The listing builds one solid part. Answer for the finished solid, in the listing's coordinates (mm). A direction names the side the tool comes from. Round coordinates to 2 decimals unless told otherwise and drop trailing zeros. Write each loop counter-clockwise with the first axis right and the second up, starting at its lowest first coordinate (ties: lowest second). Pieces come first, ordered by that corner, then holes.
from build123d import *

# Parameters (mm, degrees)
EXTRUDE1_DEPTH  = 4.7752
EXTRUDE2_DEPTH  = 12.938
SKETCH33_W      = 2.286
SKETCH33_H      = 5.588
EXTRUDE30_DEPTH = 10.668
EXTRUDE3_DEPTH  = 3.0988
EXTRUDE6_DEPTH  = 3.0988
EXTRUDE7_DEPTH  = 3.0988
SKETCH23_W      = 3.0988
SKETCH23_H      = 1.133450424
EXTRUDE20_DEPTH = 2.54
EXTRUDE16_DEPTH = 3.0988
FILLET1_R       = 0.762
EXTRUDE21_DEPTH = 3.0988
FILLET2_R       = 0.762
EXTRUDE28_DEPTH = 8.0612
EXTRUDE29_REACH = 9.061
FILLET3_R       = 0.762
FILLET4_R       = 0.508
FILLET5_R       = 0.508
FILLET6_R       = 0.508
SKETCH35_R      = 1.016
EXTRUDE32_DEPTH = 8.0612


with BuildPart() as part:
    # Sketch1 → Extrude1 (new body)
    with BuildSketch(Plane.XY):
        Polygon((-14.859, 11.938), (0, 11.938), (0, 4.572), (-3.175, 4.572), (-3.175, 0), (-14.859, 0), align=None)
    extrude(amount=-EXTRUDE1_DEPTH)

    # Sketch2 → Extrude2 (cut, through all)
    with BuildSketch(Plane(origin=(0, 11.938, 0), x_dir=(1, 0, 0), z_dir=(0, 1, 0))):
        Polygon((0, 0.5842), (-4.191, 4.7752), (0, 4.7752), align=None)
    extrude(amount=-EXTRUDE2_DEPTH, mode=Mode.SUBTRACT)

    # Sketch33 → Extrude30 (add)
    with BuildSketch(Plane.ZY.offset(14.859)):
        with Locations((-5.9182, 9.144)):
            Rectangle(SKETCH33_W, SKETCH33_H)
    extrude(amount=-EXTRUDE30_DEPTH)

    # Sketch5 → Extrude3 (cut)
    with BuildSketch(Plane.XY):
        with BuildLine():
            Line((-14.859, 8.121520088), (-14.859, 0))
            Line((-14.859, 0), (-8.374207602, 0))
            ThreePointArc((-8.374207602, 0), (-5.258197931, 4.182323512), (-8.261178378, 8.44652973))
            ThreePointArc((-8.261178378, 8.44652973), (-10.099280239, 8.911418564), (-11.9888, 9.0678))
            ThreePointArc((-11.9888, 9.0678), (-13.499883528, 8.825128765), (-14.859, 8.121520088))
        make_face()
    extrude(amount=-EXTRUDE3_DEPTH, mode=Mode.SUBTRACT)

    # Sketch8 → Extrude6 (add)
    with BuildSketch(Plane.XY):
        with BuildLine():
            Line((-5.916117419, 6.569687461), (-7.995771884, 6.569687461))
            ThreePointArc((-7.995771884, 6.569687461), (-8.381805974, 7.063274265), (-8.837117419, 7.493787609))
            Line((-8.837117419, 7.493787609), (-8.837117419, 8.601687461))
            ThreePointArc((-8.837117419, 8.601687461), (-7.16441835, 7.890723622), (-5.916117419, 6.569687461))
        make_face()
    extrude(amount=-EXTRUDE6_DEPTH)

    # Sketch9 → Extrude7 (add)
    with BuildSketch(Plane.XY):
        with BuildLine():
            Line((-5.916117419, 1.913912539), (-7.995771884, 1.913912539))
            ThreePointArc((-7.995771884, 1.913912539), (-8.381805974, 1.420325735), (-8.837117419, 0.989812391))
            Line((-8.837117419, 0.989812391), (-8.837117419, 0))
            Line((-8.837117419, 0), (-8.374207602, 0))
            ThreePointArc((-8.374207602, 0), (-6.971998867, 0.734557469), (-5.916117419, 1.913912539))
        make_face()
    extrude(amount=-EXTRUDE7_DEPTH)

    # Sketch23 → Extrude20 (add)
    with BuildSketch(Plane.ZY.offset(8.837117419)):
        with Locations((-1.5494, 8.060512821)):
            Rectangle(SKETCH23_W, SKETCH23_H)
    extrude(amount=-EXTRUDE20_DEPTH)

    # Sketch18 → Extrude16 (cut)
    with BuildSketch(Plane.XY):
        with BuildLine():
            Line((-4.903581733, 6.569687461), (-5.916117419, 6.569687461))
            ThreePointArc((-5.916117419, 6.569687461), (-5.2578, 4.2418), (-5.916117419, 1.913912539))
            Line((-5.916117419, 1.913912539), (-4.903581733, 1.913912539))
            ThreePointArc((-4.903581733, 1.913912539), (-4.3688, 4.2418), (-4.903581733, 6.569687461))
        make_face()
    extrude(amount=-EXTRUDE16_DEPTH, mode=Mode.SUBTRACT)

    # Fillet1
    fillet1_edges = [part.edges().sort_by_distance(p)[0] for p in [
        (0, 8.255, -0.5842),
    ]]
    fillet(fillet1_edges, radius=FILLET1_R)

    # Sketch24 → Extrude21 (add)
    with BuildSketch(Plane.XY):
        with BuildLine():
            Line((-8.837117419, 7.493787609), (-9.830149409, 8.301066631))
            ThreePointArc((-9.830149409, 8.301066631), (-10.843412246, 8.870424655), (-11.9888, 9.0678))
            Line((-11.9888, 9.0678), (-8.837117419, 9.0678))
            Line((-8.837117419, 9.0678), (-8.837117419, 7.493787609))
        make_face()
    extrude(amount=-EXTRUDE21_DEPTH)

    # Fillet2
    fillet2_edges = [part.edges().sort_by_distance(p)[0] for p in [
        (-14.859, 0, -3.937),
    ]]
    fillet(fillet2_edges, radius=FILLET2_R)

    # Sketch31 → Extrude28 (cut, through all)
    with BuildSketch(Plane.XY):
        Polygon((-3.175, 1.499352844), (-4.224858164, 0), (-3.175, 0), align=None)
    extrude(amount=-EXTRUDE28_DEPTH, mode=Mode.SUBTRACT)

    # Extrude29: up to this face of the body (flat: up to its plane)
    extrude29_end = Plane(part.part.faces().sort_by_distance((-2.383005057, 7.601249614, -2.967205057))[0])
    # Sketch32 → Extrude29 (add, up to the picked face)
    with BuildSketch(Plane.XY, mode=Mode.PRIVATE) as extrude29_sk1:
        Polygon((-3.175, 1.499352844), (-2.159, 2.950351219), (-2.159, 4.572), (-3.175, 4.572), align=None)
    extrude29_tool1 = split(extrude(extrude29_sk1.sketch, amount=-EXTRUDE29_REACH, mode=Mode.PRIVATE), bisect_by=extrude29_end, keep=Keep.BOTH, mode=Mode.PRIVATE)
    add(extrude29_tool1.solids().sort_by_distance((-2.719341, 3.361051, 0))[0])

    # Fillet3
    fillet3_edges = [part.edges().sort_by_distance(p)[0] for p in [
        (-4.224858164, 0, -2.3876),
    ]]
    fillet(fillet3_edges, radius=FILLET3_R)

    # Fillet4
    fillet4_edges = [part.edges().sort_by_distance(p)[0] for p in [
        (-3.078168199, 1.637642987, 0),
        (-4.269677813, 0.086097745, 0),
        (-6.729323838, 0, 0),
    ]]
    fillet(fillet4_edges, radius=FILLET4_R)

    # Fillet5
    fillet5_edges = [part.edges().sort_by_distance(p)[0] for p in [
        (-9.525, 11.938, -7.0612),
        (-9.525, 6.35, -7.0612),
        (-7.4295, 11.938, 0),
        (-14.859, 11.938, -3.5306),
    ]]
    fillet(fillet5_edges, radius=FILLET5_R)

    # Fillet6
    fillet6_edges = [part.edges().sort_by_distance(p)[0] for p in [
        (-7.995771884, 6.569687461, -1.5494),
        (-8.837117419, 0.989812391, -1.5494),
        (-7.995771884, 1.913912539, -1.5494),
    ]]
    fillet(fillet6_edges, radius=FILLET6_R)

    # Sketch35 → Extrude32 (cut, through all)
    with BuildSketch(Plane.XY):
        with Locations((-6.731, 8.763)):
            Circle(SKETCH35_R)
    extrude(amount=-EXTRUDE32_DEPTH, mode=Mode.SUBTRACT)


solid = part.part
1. Section D-D on x = -11 is taken. Determine the outline of the cut face in (y, z), plus the area to 3 significant figures.
Geometry says:
outline: (0, -4.78) - (6.35, -4.78) - (6.35, -6.55) arc R0.51 ccw to (6.86, -7.06) - (11.43, -7.06) arc R0.51 ccw to (11.94, -6.55) - (11.94, -0.51) arc R0.51 ccw to (11.43, 0) - (8.92, 0) - (8.92, -3.1) - (0, -3.1) - close
area: 42.0 mm2
2. For a pull along X with two mould halves and no side action, classify faces 1 (the face through (-2.179, 7.43, -2.764)), 2 (the face through (-9, 11.938, -4)), 3 (the face through (-13.48, 8.83, -1.53)) as released by +X, released by -X, zero draft, split by the parting line, or undercut.
Geometry says:
face 1: released by +X
face 2: zero draft
face 3: undercut
3. Section A-A on z = -4.25 is taken. Determine the outline of the cut face in (x, y) (3 decimals).
Geometry says:
outline: (-14.859, 0.762) arc R0.762 ccw to (-14.097, 0) - (-4.622, 0) arc R0.762 ccw to (-3.997, 0.325) - (-3.666, 0.798) - (-3.666, 11.938) - (-14.351, 11.938) arc R0.508 ccw to (-14.859, 11.43) - close; hole circle Ø2.032 at (-6.731, 8.763)
4. Section B-B on y = 10.5 is taken. Determine the outline of the cut face in (x, z), plus the area to 3 significant figures.
Geometry says:
outline: (-14.86, -7.06) - (-4.19, -7.06) - (-4.19, -4.78) - (-0.22, -0.81) arc R0.76 ccw to (0, -0.27) - (0, 0) - (-14.86, 0) - close
area: 86.5 mm2
5. Straight lines are drawn through the part: line 1 along Y through (x, z) = (-11.25, -5); line 2 along X through (y, z) = (10, -6.25); line 3 along X through (y, z) = (8, -4.25). For each, find the intervals that lie inside material, in ascending order.
Geometry says:
line 1: y = 6.35 to 11.94
line 2: x = -14.86 to -4.19
line 3: x = -14.86 to -7.4, -6.06 to -3.67
6. Given pin 1 (2.5 mm diameter, centred on y = 8, z = -5.5, fed in from +X); pin 2 (1.6 mm diameter, centred on x = -6.731, y = 8.763, fed in from -Z); pin 3 (3 mm diameter, centred on x = -1.5, y = 9, fed in from +Z); pin 4 (1 mm diameter, centred on y = 6, z = -3, fed in from +X), each flat-ended and moving along its own axis, determine where each tip first touches the part or whether it passes through.
Geometry says:
pin 1: stops at x = -3.67
pin 2: passes through
pin 3: stops at z = 0
pin 4: stops at x = -1.92
7. A tool of negligible diameter and unlimited length cuts with its end or side. For faces 4 (the face through (-6, 1.914, -2)), 5 (the face through (-1, 4.572, -1)), 6 (the face through (-9.327, 7.892, -1.528)), 7 (the face through (-4.191, 9, -6)), 8 (the face through (-9, 3, -4.775)), from which of +Z, -Z, +X, -X, +Y, -Y can it reach the whole face along a straight path? Write none if from no direction.
Geometry says:
face 4: +Z, -X
face 5: +Z, -Z, +X, -Y
face 6: +Z, -Y
face 7: -Z, +X, +Y, -Y
face 8: -Z, +X, -X, -Y
8. Section C-C on x = -7.5 is taken. Determine the outline of the cut face in (y, z).
Geometry says:
outline: (0, -4.78) - (6.35, -4.78) - (6.35, -6.55) arc R0.51 ccw to (6.86, -7.06) - (8.1, -7.06) - (8.1, 0) - (6.57, 0) - (6.57, -3.1) - (1.91, -3.1) - (1.91, 0) - (0.51, 0) arc R0.51 ccw to (0, -0.51) - close; (9.43, -7.06) - (11.43, -7.06) arc R0.51 ccw to (11.94, -6.55) - (11.94, -0.51) arc R0.51 ccw to (11.43, 0) - (9.43, 0) - close
